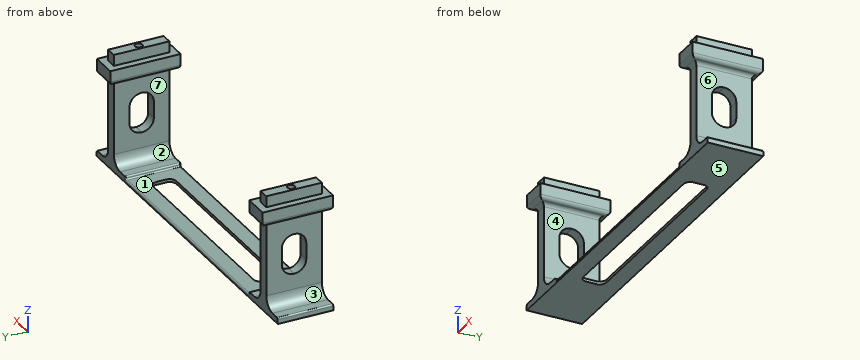
from build123d import *

# Parameters (mm, degrees)
SKETCH1_W           = 65
SKETCH1_H           = 15
BOSS_EXTRUDE1_DEPTH = 0.8
SKETCH1_3_W         = 6
SKETCH1_3_H         = 15
BOSS_EXTRUDE2_DEPTH = 1.6
BOSS_EXTRUDE3_DEPTH = 29
SKETCH2_W           = 7
SKETCH2_H           = 19
SKETCH2_W_2         = 3
SKETCH2_H_2         = 15
BOSS_EXTRUDE4_DEPTH = 4
SKETCH2_2_W         = 3
SKETCH2_2_H         = 15
BOSS_EXTRUDE5_DEPTH = 3
SKETCH3_R           = 1
CUT_EXTRUDE1_DEPTH  = 4.6
FILLET1_R           = 3.2
FILLET2_R           = 0.4
FILLET3_R           = 1
SKETCH4_W           = 56.2
SKETCH4_H           = 6.2
CUT_EXTRUDE2_DEPTH  = 64.705737631
FILLET4_R           = 1.8
SKETCH5_W           = 10.8
SKETCH5_H           = 6.6
CUT_EXTRUDE3_DEPTH  = 98.437864541
FILLET5_R           = 3.2


with BuildPart() as part:
    # Sketch1 → Boss-Extrude1 (new body)
    with BuildSketch(Plane.XY):
        with Locations((2.857159974, 13.933681879)):
            Rectangle(SKETCH1_W, SKETCH1_H)
    extrude(amount=BOSS_EXTRUDE1_DEPTH)

    # Sketch1<3> → Boss-Extrude2 (add)
    with BuildSketch(Plane.XY):
        with Locations((-32.642840026, 13.933681879)):
            Rectangle(SKETCH1_3_W, SKETCH1_3_H)
        with Locations((-41.642840026, 13.933681879)):
            Rectangle(SKETCH1_3_W, SKETCH1_3_H)
        with Locations((38.357159974, 13.933681879)):
            Rectangle(SKETCH1_3_W, SKETCH1_3_H)
        with Locations((47.357159974, 13.933681879)):
            Rectangle(SKETCH1_3_W, SKETCH1_3_H)
    extrude(amount=BOSS_EXTRUDE2_DEPTH)


with BuildPart() as boss_extrude2_piece_1:
    # of the separate pieces the step leaves, piece 1, a body of its own (boss_extrude2_pieces)
    add(part.part.solids().sort_by_distance((41.357159974, 21.433681879, 0))[0])



with BuildPart() as boss_extrude2_piece_2:
    # of the separate pieces the step leaves, piece 2, a body of its own (boss_extrude2_pieces)
    add(part.part.solids().sort_by_distance((50.357159974, 6.433681879, 0))[0])


with BuildPart() as boss_extrude2_piece_3:
    # of the separate pieces the step leaves, piece 3, a body of its own (boss_extrude2_pieces)
    add(part.part.solids().sort_by_distance((-38.642840026, 6.433681879, 0))[0])


with BuildPart() as boss_extrude2_piece_1_1:
    add(boss_extrude2_piece_1.part)

    add(boss_extrude2_piece_2.part)  # Boss-Extrude3 merges Boss-Extrude2 piece 2

    add(boss_extrude2_piece_3.part)  # Boss-Extrude3 merges Boss-Extrude2 piece 3
    # Sketch1<4> → Boss-Extrude3 (add)
    with BuildSketch(Plane.XY):
        Polygon((-35.642840026, 6.433681879), (-35.642840026, 21.433681879), (-37.142840026, 21.433681879), (-38.642840026, 21.433681879), (-38.642840026, 6.433681879), (-37.142840026, 6.433681879), align=None)
        Polygon((42.857159974, 21.433681879), (41.357159974, 21.433681879), (41.357159974, 6.433681879), (42.857159974, 6.433681879), (44.357159974, 6.433681879), (44.357159974, 21.433681879), align=None)
    extrude(amount=BOSS_EXTRUDE3_DEPTH)

    # Sketch2 → Boss-Extrude4 (add)
    # profile 1 of 2: a face of its own
    with BuildSketch(Plane.XY.offset(29)):
        with Locations((-37.142840026, 13.933681879)):
            Rectangle(SKETCH2_W, SKETCH2_H)
        with Locations((-37.142840026, 13.933681879)):
            Rectangle(SKETCH2_W_2, SKETCH2_H_2, mode=Mode.SUBTRACT)
    # profile 2 of 2: a face of its own
    with BuildSketch(Plane.XY.offset(29)):
        with Locations((42.857159974, 13.933681879)):
            Rectangle(SKETCH2_W, SKETCH2_H)
        with Locations((42.857159974, 13.933681879)):
            Rectangle(SKETCH2_W_2, SKETCH2_H_2, mode=Mode.SUBTRACT)
    extrude(amount=-BOSS_EXTRUDE4_DEPTH)

    # Sketch2<2> → Boss-Extrude5 (add)
    with BuildSketch(Plane.XY.offset(29)):
        with Locations((-37.142840026, 13.933681879)):
            Rectangle(SKETCH2_2_W, SKETCH2_2_H)
        with Locations((42.857159974, 13.933681879)):
            Rectangle(SKETCH2_2_W, SKETCH2_2_H)
    extrude(amount=BOSS_EXTRUDE5_DEPTH)

    # Sketch3 → Cut-Extrude1 (cut)
    with BuildSketch(Plane.XY.offset(32)):
        with Locations((-37.142840026, 13.933681879)):
            Circle(SKETCH3_R)
        with Locations((42.857159974, 13.933681879)):
            Circle(SKETCH3_R)
    extrude(amount=-CUT_EXTRUDE1_DEPTH, mode=Mode.SUBTRACT)

    # Fillet1
    fillet1_edges = [boss_extrude2_piece_1_1.edges().sort_by_distance(p)[0] for p in [
        (44.357159974, 13.933681879, 1.6),
        (41.357159974, 13.933681879, 1.6),
        (-35.642840026, 13.933681879, 1.6),
        (-38.642840026, 13.933681879, 1.6),
    ]]
    fillet(fillet1_edges, radius=FILLET1_R)

    # Fillet2
    fillet2_edges = [boss_extrude2_piece_1_1.edges().sort_by_distance(p)[0] for p in [
        (-29.642840026, 21.433681879, 1.2),
        (35.357159974, 21.433681879, 1.2),
        (-29.642840026, 6.433681879, 1.2),
        (35.357159974, 6.433681879, 1.2),
        (2.857159974, 21.433681879, 0.8),
        (2.857159974, 6.433681879, 0.8),
        (50.357159974, 13.933681879, 1.6),
        (35.357159974, 13.933681879, 0.8),
        (35.357159974, 13.933681879, 1.6),
        (-29.642840026, 13.933681879, 0.8),
        (-29.642840026, 13.933681879, 1.6),
        (-44.642840026, 13.933681879, 1.6),
    ]]
    fillet(fillet2_edges, radius=FILLET2_R - 0.0001)  # a hair under: the kernel refuses the full size

    # Fillet3
    fillet3_edges = [boss_extrude2_piece_1_1.edges().sort_by_distance(p)[0] for p in [
        (-37.142840026, 23.433681879, 25),
        (-40.642840026, 13.933681879, 25),
        (-33.642840026, 13.933681879, 25),
        (-37.142840026, 4.433681879, 25),
        (42.857159974, 23.433681879, 25),
        (39.357159974, 13.933681879, 25),
        (42.857159974, 4.433681879, 25),
        (46.357159974, 13.933681879, 25),
        (42.857159974, 6.433681879, 25),
        (41.357159974, 13.933681879, 25),
        (42.857159974, 21.433681879, 25),
        (44.357159974, 13.933681879, 25),
        (-37.142840026, 21.433681879, 25),
        (-35.642840026, 13.933681879, 25),
        (-37.142840026, 6.433681879, 25),
        (-38.642840026, 13.933681879, 25),
    ]]
    fillet(fillet3_edges, radius=FILLET3_R - 0.0001)  # a hair under: the kernel refuses the full size

    # Sketch4 → Cut-Extrude2 (cut, through all)
    with BuildSketch(Plane.XY.offset(0.8)):
        with Locations((2.857159974, 13.933681879)):
            Rectangle(SKETCH4_W, SKETCH4_H)
    extrude(amount=-CUT_EXTRUDE2_DEPTH, mode=Mode.SUBTRACT)

    # Fillet4
    fillet4_edges = [boss_extrude2_piece_1_1.edges().sort_by_distance(p)[0] for p in [
        (30.957159974, 10.833681879, 0.4),
        (-25.242840026, 10.833681879, 0.4),
        (-25.242840026, 17.033681879, 0.4),
        (30.957159974, 17.033681879, 0.4),
    ]]
    fillet(fillet4_edges, radius=FILLET4_R)

    # Sketch5 → Cut-Extrude3 (cut, through all)
    with BuildSketch(Plane(origin=(44.357159974, 0, 0), x_dir=(0, 0, -1), z_dir=(1, 0, 0))):
        with Locations((-14.4, 13.933681879)):
            Rectangle(SKETCH5_W, SKETCH5_H)
    extrude(amount=-CUT_EXTRUDE3_DEPTH, mode=Mode.SUBTRACT)

    # Fillet5
    fillet5_edges = [boss_extrude2_piece_1_1.edges().sort_by_distance(p)[0] for p in [
        (-37.142840026, 17.233681879, 9),
        (42.857159974, 17.233681879, 9),
        (-37.142840026, 10.633681879, 9),
        (42.857159974, 10.633681879, 9),
        (-37.142840026, 10.633681879, 19.8),
        (42.857159974, 10.633681879, 19.8),
        (-37.142840026, 17.233681879, 19.8),
        (42.857159974, 17.233681879, 19.8),
    ]]
    fillet(fillet5_edges, radius=FILLET5_R)


solid = boss_extrude2_piece_1_1.part
For this review, take the finished solid that the model builds, in its own axes (mm). Face numbers are marked on the shaded views. A direction names the side the tool comes from. Round coordinates to 2 decimals unless told otherwise and drop trailing zeros. Order: outer loops, then holes, each group sorted by start corner. A loop starts at its lowest first (then second) coordinate and runs counter-clockwise, first axis right, second up. Notation, with made-up numbers: M 13.5,66.25 L 37.5,66.25 A30 ccw 37.5,90.25 Z; hole C 47.25,12 d7. An arc over 180 degrees is marked long. Use a Markdown table: item, result. Add a question column.
Item 1: Add section A-A, the plane x = 18.5. Give the boundary of the cut face in (y, z), then the cut area to 3 significant figures.
Item 2: Add section D-D, the plane z = 3. Give the boundary of the cut face in (x, y).
Item 3: Insertion check: pin 1 (4.5 mm diameter, centred on y = 10.5, z = 17.5, fed in from +X); pin 2 (3.5 mm diameter, centred on x = -36.5, z = 31, fed in from -Y); pin 3 (6 mm diameter, centred on x = -4.5, y = 14.5, fed in from -Z); pin 4 (0.9 mm diameter, centred on x = -37.5, z = 30.5, fed in from +Y). Each pin has a flat end and moves straight along its axis. Give the tip position at first contact, or say it passes through.
Item 4: Add section C-C, the plane z = 17.5. Give the boundary of the cut face in (x, y).
Item 5: To check wall thickness, follow line 1 along X through (y, z) = (12.5, 26); line 2 along X through (y, z) = (21, 14.5); line 3 along Z through (x, y) = (-28, 19.75). State the ranges of each line that lie inside material, in increasing order.
Item 6: Add section B-B, the plane z = 23. Give the boundary of the cut face in (x, y).
Item 7: Mouldability with a two-part tool opening along X and no side actions: class the marked faces 4, 5, 6 and 7 as released by +X, released by -X, zero draft, split by the parting line, or undercut.
Item 8: Tool access review of the marked faces 1, 2 and 3: name each direction out of +Z, -Z, +X, -X, +Y, -Y from which nothing blocks a thin tool from reaching the whole face with its end or side.
Geometry results:
| question | item | result |
|---|---|---|
| 1 | outline | M 6.43,0 L 10.83,0 L 10.83,0.8 L 6.83,0.8 A0.4 ccw 6.43,0.4 Z; M 17.03,0 L 21.43,0 L 21.43,0.4 A0.4 ccw 21.03,0.8 L 17.03,0.8 Z |
| 1 | area | 6.97 mm² |
| 2 | outline | M -39.2,6.43 L -35.09,6.43 L -35.09,21.43 L -39.2,21.43 Z; M 40.8,6.43 L 44.91,6.43 L 44.91,21.43 L 40.8,21.43 Z |
| 3 | pin 1 | stops at x = 44.36 |
| 3 | pin 2 | stops at y = 6.43 |
| 3 | pin 3 | stops at z = 0 |
| 3 | pin 4 | stops at y = 21.43 |
| 4 | outline | M -38.64,6.43 L -35.64,6.43 L -35.64,10.76 L -38.64,10.76 Z; M -38.64,17.1 L -35.64,17.1 L -35.64,21.43 L -38.64,21.43 Z; M 41.36,6.43 L 44.36,6.43 L 44.36,10.76 L 41.36,10.76 Z; M 41.36,17.1 L 44.36,17.1 L 44.36,21.43 L 41.36,21.43 Z |
| 5 | line 1 | x = -40.64 to -33.64, 39.36 to 46.36 |
| 5 | line 2 | x = -38.64 to -35.64, 41.36 to 44.36 |
| 5 | line 3 | z = 0 to 0.8 |
| 6 | outline | M -38.64,6.43 L -35.64,6.43 L -35.64,21.43 L -38.64,21.43 Z; M 41.36,6.43 L 44.36,6.43 L 44.36,21.43 L 41.36,21.43 Z |
| 7 | face 4 | undercut |
| 7 | face 5 | zero draft |
| 7 | face 6 | released by +X |
| 7 | face 7 | undercut |
| 8 | face 1 | +Z, +Y, -Y |
| 8 | face 2 | +Y, -Y |
| 8 | face 3 | -X, +Y, -Y |
